Geometry check sheet. Reference: the model listing, model coordinates, mm. Face numbers are marked on the shaded views. A direction names the side the tool comes from. Coordinates: 2 decimals unless noted, no trailing zeros. Write each loop counter-clockwise with the first axis right and the second up, starting at its lowest first coordinate (ties: lowest second). Pieces come first, ordered by that corner, then holes. Notation, with made-up numbers: (-19, 74) -> (-13, 74) arc R22 ccw to (-13, 96) -> close; hole circle Ø9 at (38.5, 84). An arc over 180 degrees is marked (long way). Answer in a Markdown table with one row per item. Add a question column.
Q1. Section check A-A, the plane z = 1.5. Record the boundary of the cut face in (x, y).
Q2. Release check for a two-part mould opening along Y. For the marked faces 3, 4, 5 and 6 record: pulls with the +Y half, pulls with the -Y half, needs draft (parallel to the pull), parting line crosses it, or undercut.
Q3. Thickness scan on line 1 (X direction, y = -5, z = 52.5); line 2 (Y direction, x = -2, z = 53.5); line 3 (X direction, y = 4.5, z = 48). Record the ranges inside material, lowest first.
Q4. Section check B-B, the plane z = 12.5. Record the boundary of the cut face in (x, y) (3 decimals).
Q5. Tool access check on the marked faces 1 and 2. Record the directions out of +Z, -Z, +X, -X, +Y, -Y that give a thin tool (end or side, any length) a straight path to the whole face; none if there is none.
Q6. Section check C-C, the plane x = 9. Count the separate pieces of the cut face and the enclosed holes in it, and give its area (3 significant figures).
Q7. Gauge pin test, flat ends, axial feed: P1, Ø1.9, axis at x = 12.01, y = 12.67, coming from the +Z side; P2, Ø3, axis at x = -16, z = 20, coming from the +Y side; P3, Ø1.9, axis at x = 7, z = 31, coming from the +Y side (3 decimals); P4, Ø20, axis at x = -10, y = -5, coming from the +Z side. Record the tip position at first contact, or that the pin passes through.
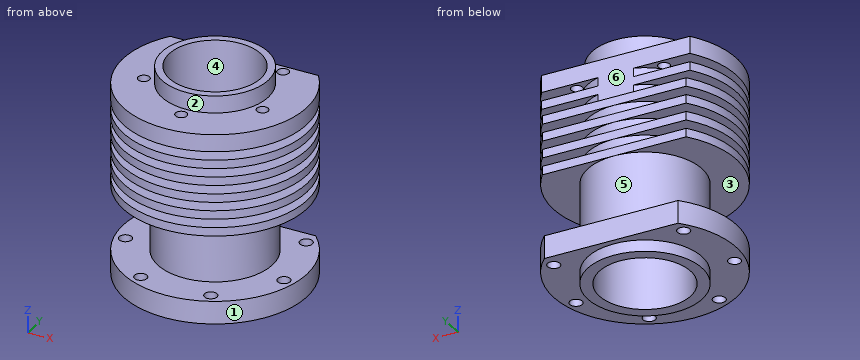
```python
from build123d import *

# Parameters (mm, degrees)
F0_R      = 25.4
F1_DEPTH  = 53.0098
F2_R      = 14.732
F3_DEPTH  = 4.7625
F4_R      = 15.875
F5_DEPTH  = 3.175
F7_R      = 12.7
F8_DEPTH  = 60.9483
F9_W      = 12.1422023922
F9_H      = 2.3622
F11_W     = 13.3322854936
F11_H     = 18.2753
F14_DEPTH = 11.8618
F16_DEPTH = 16.637
F18_DEPTH = 6.477
F20_D     = 3.4544
F20_DEPTH = 7.62
F20_TIP   = 1.0378064612
F22_D     = 3.175
F22_DEPTH = 6.35
F22_TIP   = 0.9538662327


# Not quite as in the source:
# - a feature names something its author has since deleted; it is built from what else it names


with BuildPart() as f1:
    # F0 (on Top) → F1 (new body)
    with BuildSketch(Plane.XY):
        Circle(F0_R)
    extrude(amount=F1_DEPTH)

    # F2 (on face) → F3 (join)
    with BuildSketch(Plane.XY.offset(53.0098)):
        Circle(F2_R)
    extrude(amount=F3_DEPTH)

    # F4 (on face) → F5 (join)
    with BuildSketch(Plane(origin=(0, 0, 0), x_dir=(1, 0, 0), z_dir=(0, 0, -1))):
        Circle(F4_R)
    extrude(amount=F5_DEPTH)

    # F7 (on face) → F8 (cut, through all)
    with BuildSketch(Plane(origin=(0, 0, -3.175), x_dir=(1, 0, 0), z_dir=(0, 0, -1))):
        Circle(F7_R)
    extrude(amount=-F8_DEPTH, mode=Mode.SUBTRACT)

    # F9 (on Front) → F10 (revolve, cut)
    with BuildSketch(Plane.XZ):
        with Locations((21.9461011961, 47.0662)):
            Rectangle(F9_W, F9_H)
        with Locations((21.9461011961, 42.3418)):
            Rectangle(F9_W, F9_H)
        with Locations((21.9461011961, 37.6174)):
            Rectangle(F9_W, F9_H)
        with Locations((21.9461011961, 32.893)):
            Rectangle(F9_W, F9_H)
        with Locations((21.9461011961, 28.1686)):
            Rectangle(F9_W, F9_H)
    revolve(axis=Axis((0, 0, 0), (0, 0, -1)), mode=Mode.SUBTRACT)

    # F11 (on Front) → F12 (revolve, cut)
    with BuildSketch(Plane.XZ):
        with Locations((22.5411427468, 15.48765)):
            Rectangle(F11_W, F11_H)
    revolve(axis=Axis((0, 0, 0), (0, 0, -1)), mode=Mode.SUBTRACT)

    # F13 (on face) → F14 (cut)
    with BuildSketch(Plane.XY.offset(53.0098)):
        with BuildLine():
            Line((-28.8578128478, 32.0924090841), (-28.8578128478, 15.0876))
            Line((-28.8578128478, 15.0876), (-20.4334120068, 15.0876))
            ThreePointArc((-20.4334120068, 15.0876), (0, 25.4), (20.4334120068, 15.0876))
            Line((20.4334120068, 15.0876), (35.4937171599, 15.0876))
            Line((35.4937171599, 15.0876), (35.4937171599, 32.0924090841))
            Line((35.4937171599, 32.0924090841), (-28.8578128478, 32.0924090841))
        make_face()
        with BuildLine():
            ThreePointArc((20.4334120068, 15.0876), (0, 25.4), (-20.4334120068, 15.0876))
            Line((-20.4334120068, 15.0876), (20.4334120068, 15.0876))
        make_face()
    extrude(amount=-F14_DEPTH, mode=Mode.SUBTRACT)

    # F15 (on face) → F16 (cut)
    with BuildSketch(Plane.XY.offset(41.148)):
        with BuildLine():
            Line((22.7077871409, 25.7988459408), (-23.4762642381, 25.7988459408))
            Line((-23.4762642381, 25.7988459408), (-23.4762642381, 15.875))
            Line((-23.4762642381, 15.875), (-19.8278686449, 15.875))
            ThreePointArc((-19.8278686449, 15.875), (0, 25.4), (19.8278686449, 15.875))
            Line((19.8278686449, 15.875), (22.7077871409, 15.875))
            Line((22.7077871409, 15.875), (22.7077871409, 25.7988459408))
        make_face()
        with BuildLine():
            ThreePointArc((19.8278686449, 15.875), (0, 25.4), (-19.8278686449, 15.875))
            Line((-19.8278686449, 15.875), (19.8278686449, 15.875))
        make_face()
    extrude(amount=-F16_DEPTH, mode=Mode.SUBTRACT)

    # F17 (on face) → F18 (cut)
    with BuildSketch(Plane(origin=(0, 0, 0), x_dir=(1, 0, 0), z_dir=(0, 0, -1))):
        with BuildLine():
            Line((-18.4330514283, -17.4752), (-34.0658536954, -17.4752))
            Line((-34.0658536954, -17.4752), (-34.0658536954, -39.2576220664))
            Line((-34.0658536954, -39.2576220664), (38.0722320481, -39.2576220664))
            Line((38.0722320481, -39.2576220664), (38.0722320481, -17.4752))
            Line((38.0722320481, -17.4752), (18.4330514283, -17.4752))
            ThreePointArc((18.4330514283, -17.4752), (0, -25.4), (-18.4330514283, -17.4752))
        make_face()
        with BuildLine():
            Line((18.4330514283, -17.4752), (-18.4330514283, -17.4752))
            ThreePointArc((-18.4330514283, -17.4752), (0, -25.4), (18.4330514283, -17.4752))
        make_face()
    extrude(amount=-F18_DEPTH, mode=Mode.SUBTRACT)

    # F20
    with Locations(Plane(origin=(0, 0, 0), x_dir=(1, 0, 0), z_dir=(0, 0, -1))):
        with Locations((-17.907, -13.5636), (-21.844, 5.334), (-9.652, 20.2946), (9.652, 20.2946), (21.844, 5.334), (17.907, -13.5636)):
            Hole(F20_D / 2, depth=F20_DEPTH)
            with Locations((0, 0, -(F20_DEPTH + F20_TIP / 2))):  # 118° drill point
                Cone(0, F20_D / 2, F20_TIP, mode=Mode.SUBTRACT)

    # F22
    with Locations(Plane.XY.offset(53.0098)):
        with Locations((-12.0142, 12.6746), (12.0142, 12.6746), (16.3576, -6.1214), (-16.3576, -6.1214), (0, -17.4752)):
            Hole(F22_D / 2, depth=F22_DEPTH)
            with Locations((0, 0, -(F22_DEPTH + F22_TIP / 2))):  # 118° drill point
                Cone(0, F22_D / 2, F22_TIP, mode=Mode.SUBTRACT)


solid = f1.part
```
Calculated:
| question | item | result |
|---|---|---|
| 1 | outline | (-18.43, 17.48) arc R25.4 ccw (long way) to (18.43, 17.48) -> close; hole circle Ø3.45 at (-21.84, -5.33); hole circle Ø3.45 at (-17.91, 13.56); hole circle Ø25.4 at (0, 0); hole circle Ø3.45 at (-9.65, -20.29); hole circle Ø3.45 at (9.65, -20.29); hole circle Ø3.45 at (17.91, 13.56); hole circle Ø3.45 at (21.84, -5.33) |
| 2 | face 3 | needs draft |
| 2 | face 4 | undercut |
| 2 | face 5 | parting line crosses it |
| 2 | face 6 | pulls with the +Y half |
| 3 | line 1 | x = -24.9 to -17.48, -15.23 to -11.67, 11.67 to 15.23, 17.48 to 24.9 |
| 3 | line 2 | y = -14.6 to -12.54, 12.54 to 14.6 |
| 3 | line 3 | x = -15.22 to -11.88, 11.88 to 15.22 |
| 4 | outline | circle Ø31.75 at (0, 0); hole circle Ø25.4 at (0, 0) |
| 5 | face 1 | +Z, -Z |
| 5 | face 2 | +Z |
| 6 | separate pieces | 3 |
| 6 | enclosed holes | 0 |
| 6 | area | 781 mm² |
| 7 | P1 | stops at z = 45.89 |
| 7 | P2 | stops at y = 6.46 |
| 7 | P3 | stops at y = 15.875 |
| 7 | P4 | stops at z = 57.77 |
